Part model, mm, in its own coordinate system. A direction names the side the tool comes from. Give positions to 0.01 mm unless a question says otherwise; leave off trailing zeros. Write each loop counter-clockwise with the first axis right and the second up, starting at its lowest first coordinate (ties: lowest second). Pieces come first, ordered by that corner, then holes. Notation, with made-up numbers: (55.5, 20) - (106.5, 20) arc R22 cw to (106.5, 30) - close; hole circle Ø5 at (75.5, 83). An arc over 180 degrees is marked (long way). Answer in a Markdown table with one row per item. Add a question column.
1. Drop flat-ended pins along their axis: pin 1 Ø1.2 at (x, z) = (0.5, 13.5) entering from -Y; pin 2 Ø5 at (y, z) = (119.5, -22) entering from -X; pin 3 Ø1.5 at (x, y) = (-19.5, 225) entering from -Z. Give the stop position or say it passes through.
2. Probe line 1 along X through (y, z) = (-32, 0); line 2 along Y through (x, z) = (24, -16); line 3 along Y through (x, z) = (-6, -4.5). List the from-to ranges inside material, lowest first.
3. Pull direction Z, two halves, no side cores. Call faces 1 (the flat face through (17, -43.2, -17)), 2 (the cylindrical face through (7.509, 443.986, 23.846)), 3 (the cylindrical face through (3.9, -30.3, -12.4)): released by +Z, released by -Z, zero draft, split by the parting line, or undercut.
4. Band-saw the part on B-B on y = 139. Write the cut outline in (x, z), plus the area to 3 significant figures.
5. Which spindle directions (+Z, -Z, +X, -X, +Y, -Y) get a long thin tool onto all of the face, cutting with end or side? Do faces 4 (the flat face through (-21, 400, 21)), 5 (the cylindrical face through (20.85, -41.58, -10.84)), 6 (the cylindrical face through (-7.509, -20.773, 23.846)). Say none if no direction does.
6. Band-saw the part on A-A on y = -19. Write the cut outline in (x, z), plus the area to 3 significant figures.
```python
from build123d import *

# Parameters (mm, degrees)
ESQUISSE1_R             = 50
BOSS_EXTRU_1_DEPTH      = 400
ESQUISSE2_R             = 25
BOSS_EXTRU_2_DEPTH      = 46
BOSS_EXTRU_3_START      = 50
ESQUISSE3_R             = 25
BOSS_EXTRU_3_DEPTH      = 50
CONG_1_R                = 1
ENL_V_START             = -6.2
ESQUISSE4_R             = 25
ESQUISSE4_R_2           = 23.5
ENL_V_MAT_EXTRU_1_DEPTH = 3.2
ESQUISSE6_W             = 5.249523393
ESQUISSE6_H             = 3.2
CHANFREIN1_SIZE         = 1
ESQUISSE7_R             = 13
ENL_V_MAT_EXTRU_2_DEPTH = 40
ESQUISSE8_W             = 6
ESQUISSE8_H             = 5
ENL_V_MAT_EXTRU_3_DEPTH = 38


with BuildPart() as part:
    # Esquisse1 → Boss.-Extru.1 (new body)
    with BuildSketch(Plane(origin=(0, 0, 0), x_dir=(1, 0, 0), z_dir=(0, 1, 0))):
        with Locations(Location((0, 0, 0), (0, 0, 270))):
            Circle(ESQUISSE1_R)
    extrude(amount=BOSS_EXTRU_1_DEPTH)

    # Esquisse2 → Boss.-Extru.2 (add)
    with BuildSketch(Plane(origin=(0, 400, 0), x_dir=(1, 0, 0), z_dir=(0, 1, 0))):
        with Locations(Location((0, 0, 0), (0, 0, 270))):
            Circle(ESQUISSE2_R)
    extrude(amount=BOSS_EXTRU_2_DEPTH)

    # Esquisse3 → Boss.-Extru.3 (add)
    with BuildSketch(Plane.XZ.offset(BOSS_EXTRU_3_START)):
        with Locations(Location((0, 0, 0), (0, 0, 90))):
            Circle(ESQUISSE3_R)
    extrude(amount=-BOSS_EXTRU_3_DEPTH)

    # Congé1
    cong_1_edges = [part.edges().sort_by_distance(p)[0] for p in [
        (0, 0, -50),
        (0, 400, -50),
        (0, 400, -25),
        (0, 0, -25),
    ]]
    fillet(cong_1_edges, radius=CONG_1_R)

    # Esquisse4 → Enlèv. mat.-Extru.1 (cut)
    with BuildSketch(Plane(origin=(0, 446, 0), x_dir=(1, 0, 0), z_dir=(0, 1, 0)).offset(ENL_V_START)):
        with Locations(Location((0, 0, 0), (0, 0, 270))):
            Circle(ESQUISSE4_R)
        with Locations(Location((0, 0, 0), (0, 0, 270))):
            Circle(ESQUISSE4_R_2, mode=Mode.SUBTRACT)
    extrude(amount=ENL_V_MAT_EXTRU_1_DEPTH, mode=Mode.SUBTRACT)

    # Esquisse6 → Enlèvement de matière-Révolution1 (revolve, cut)
    with BuildSketch(Plane.XY, mode=Mode.PRIVATE) as enl_vement_de_mati_re_r_volution1_sk:
        with Locations((26.124761697, -41.6)):
            Rectangle(ESQUISSE6_W, ESQUISSE6_H)
    revolve(enl_vement_de_mati_re_r_volution1_sk.sketch.rotate(Axis((0, -50, 0), (0, 1, 0)), 90), axis=Axis((0, -50, 0), (0, 1, 0)), mode=Mode.SUBTRACT)

    # Chanfrein1
    chanfrein1_edges = [part.edges().sort_by_distance(p)[0] for p in [
        (0, -50, -25),
        (0, 446, -25),
    ]]
    chamfer(chanfrein1_edges, length=CHANFREIN1_SIZE)

    # Esquisse7 → Enlèv. mat.-Extru.2 (cut)
    with BuildSketch(Plane.XZ.offset(50)):
        with Locations(Location((0, 0, 0), (0, 0, 270))):
            Circle(ESQUISSE7_R)
    extrude(amount=-ENL_V_MAT_EXTRU_2_DEPTH, mode=Mode.SUBTRACT)

    # Esquisse8 → Enlèv. mat.-Extru.3 (cut)
    with BuildSketch(Plane.XZ.offset(50)):
        with Locations((0, 12.5)):
            Rectangle(ESQUISSE8_W, ESQUISSE8_H)
    extrude(amount=-ENL_V_MAT_EXTRU_3_DEPTH, mode=Mode.SUBTRACT)


solid = part.part
```
Values:
| question | item | result |
|---|---|---|
| 1 | pin 1 | stops at y = -12 |
| 1 | pin 2 | stops at x = -46.04 |
| 1 | pin 3 | stops at z = -46.35 |
| 2 | line 1 | x = -25 to -13, 13 to 25 |
| 2 | line 2 | y = 0 to 400 |
| 2 | line 3 | y = -10 to 446 |
| 3 | face 1 | zero draft |
| 3 | face 2 | split by the parting line |
| 3 | face 3 | undercut |
| 4 | outline | circle Ø100 at (0, 0) |
| 4 | area | 7,850 mm² |
| 5 | face 4 | +Y |
| 5 | face 5 | none |
| 5 | face 6 | -Y |
| 6 | outline | circle Ø50 at (0, 0); hole (-3, 12.65) arc R13 ccw (long way) to (3, 12.65) - (3, 15) - (-3, 15) - close |
| 6 | area | 1,420 mm² |
